from build123d import *

# Parameters (mm, degrees)
SKETCH2_R           = 56.35625
BOSS_EXTRUDE1_DEPTH = 25.4
SKETCH3_R           = 63.5
BOSS_EXTRUDE2_DEPTH = 9.525
SKETCH4_R           = 44.45
CUT_EXTRUDE1_DEPTH  = 97.35484225
SKETCH9_W           = 5.08
SKETCH9_H           = 12.7
FILLET1_R           = 2.54
SKETCH10_R          = 2.54
CUT_EXTRUDE2_DEPTH  = 94.3255592
CIRPATTERN1_COUNT   = 12
HOLE2_START         = 30.099
HOLE2_OUTLINE_R     = 2.413
HOLE2_DEPTH         = 4.826
HOLE2_START_2       = 25.485046345
HOLE2_2_OUTLINE_R   = 1.143
HOLE2_2_DEPTH       = 4.613953655
CIRPATTERN2_COUNT   = 2
HOLE3_D             = 2.286
HOLE3_DEPTH         = 9.438944644
HOLE3_CBORE_D       = 4.826
HOLE3_CBORE_DEPTH   = 4.826
CIRPATTERN3_COUNT   = 2


# Read off the part's stored shape, not the designer's step: Hole2
with BuildPart() as part:
    # Sketch2 → Boss-Extrude1 (new body)
    with BuildSketch(Plane(origin=(0, 0, 0), x_dir=(1, 0, 0), z_dir=(0, 1, 0))):
        with Locations(Location((0, 0, 0), (0, 0, 270))):
            Circle(SKETCH2_R)
    extrude(amount=BOSS_EXTRUDE1_DEPTH)

    # Sketch3 → Boss-Extrude2 (add)
    with BuildSketch(Plane(origin=(0, 25.4, 0), x_dir=(1, 0, 0), z_dir=(0, 1, 0))):
        with Locations(Location((0, 0, 0), (0, 0, 90))):
            Circle(SKETCH3_R)
    extrude(amount=BOSS_EXTRUDE2_DEPTH)

    # Sketch4 → Cut-Extrude1 (cut, through all)
    with BuildSketch(Plane.XZ):
        with Locations(Location((0, 0, 0), (0, 0, 270))):
            Circle(SKETCH4_R)
    extrude(amount=-CUT_EXTRUDE1_DEPTH, mode=Mode.SUBTRACT)

    # Sketch9 → Cut-Revolve1 (revolve, cut)
    with BuildSketch(Plane(origin=(0, 0, 0), x_dir=(0, 0, -1), z_dir=(1, 0, 0))):
        with Locations((53.81625, 19.05)):
            Rectangle(SKETCH9_W, SKETCH9_H)
    revolve(axis=Axis((0, 0, 0), (0, 1, 0)), mode=Mode.SUBTRACT)

    # Fillet1
    fillet1_edges = [part.edges().sort_by_distance(p)[0] for p in [
        (0, 12.7, 51.27625),
        (0, 25.4, 51.27625),
    ]]
    fillet(fillet1_edges, radius=FILLET1_R)

    # Sketch10 → Cut-Extrude2 (cut, through all)
    with BuildSketch(Plane.XZ.offset(-25.4)):
        with Locations(Location((58.42, 0, 0), (0, 0, 270))):
            Circle(SKETCH10_R)
        with Locations(Location((50.593204089, -29.21, 0), (0, 0, 270))):
            Circle(SKETCH10_R)
        with Locations(Location((29.21, -50.593204089, 0), (0, 0, 270))):
            Circle(SKETCH10_R)
        with Locations(Location((0, -58.42, 0), (0, 0, 270))):
            Circle(SKETCH10_R)
        with Locations(Location((-29.21, -50.593204089, 0), (0, 0, 270))):
            Circle(SKETCH10_R)
        with Locations(Location((-50.593204089, -29.21, 0), (0, 0, 270))):
            Circle(SKETCH10_R)
        with Locations(Location((-58.42, 0, 0), (0, 0, 270))):
            Circle(SKETCH10_R)
        with Locations(Location((-50.593204089, 29.21, 0), (0, 0, 270))):
            Circle(SKETCH10_R)
        with Locations(Location((-29.21, 50.593204089, 0), (0, 0, 270))):
            Circle(SKETCH10_R)
        with Locations(Location((0, 58.42, 0), (0, 0, 270))):
            Circle(SKETCH10_R)
        with Locations(Location((29.21, 50.593204089, 0), (0, 0, 270))):
            Circle(SKETCH10_R)
        with Locations(Location((50.593204089, 29.21, 0), (0, 0, 270))):
            Circle(SKETCH10_R)
    extrude(amount=-CUT_EXTRUDE2_DEPTH, mode=Mode.SUBTRACT)

    # Sketch12 → #10-32 Tapped Hole1 (revolve, cut)
    with BuildSketch(Plane(origin=(51.562, 0, 0), x_dir=(0, 0, -1), z_dir=(1, 0, 0))):
        Polygon((0, 0), (0, 10.103317848), (2.0193, 8.89), (2.0193, 1.0287), (3.048, 0), align=None)
    f_10_32_tapped_hole1 = revolve(axis=Axis((51.562, -6.35, 0), (0, 1, 0)), mode=Mode.SUBTRACT)

    # CirPattern1: #10-32 Tapped Hole1 ×12 about axis
    cirpattern1_axis = Axis((0, 0, 0), (0, 1, 0))
    for i in range(1, CIRPATTERN1_COUNT):
        add(f_10_32_tapped_hole1.rotate(cirpattern1_axis, i * 360 / CIRPATTERN1_COUNT), mode=Mode.SUBTRACT)

    # Hole2 outline → Hole2 (cut)
    with BuildSketch(Plane(origin=(0, 0, 0), x_dir=(1, 0, 0), z_dir=(0, 1, 0)).offset(HOLE2_START)):
        with Locations((56.429386772, -15.120208615)):
            Circle(HOLE2_OUTLINE_R)
    hole2 = extrude(amount=HOLE2_DEPTH, mode=Mode.SUBTRACT)

    # Hole2 2 outline → Hole2 2 (cut)
    with BuildSketch(Plane(origin=(0, 0, 0), x_dir=(1, 0, 0), z_dir=(0, 1, 0)).offset(HOLE2_START_2)):
        with Locations((56.429386772, -15.120208615)):
            Circle(HOLE2_2_OUTLINE_R)
    hole2_2 = extrude(amount=HOLE2_2_DEPTH, mode=Mode.SUBTRACT)

    # CirPattern2: Hole2, Hole2 2 ×2 about axis
    cirpattern2_axis = Axis((0, 0, 0), (0, 1, 0))
    add([hole2.rotate(cirpattern2_axis, i * 360 / CIRPATTERN2_COUNT) for i in range(1, CIRPATTERN2_COUNT)], mode=Mode.SUBTRACT)
    add([hole2_2.rotate(cirpattern2_axis, i * 360 / CIRPATTERN2_COUNT) for i in range(1, CIRPATTERN2_COUNT)], mode=Mode.SUBTRACT)

    # Hole3
    with Locations(Plane(origin=(0, 0, 0), x_dir=(-1, 0, 0), z_dir=(0, -1, 0))):
        with Locations((-13.345227604, -49.805067455)):
            hole3 = CounterBoreHole(HOLE3_D / 2, HOLE3_CBORE_D / 2, HOLE3_CBORE_DEPTH, depth=HOLE3_DEPTH)

    # CirPattern3: Hole3 ×2 about axis
    cirpattern3_axis = Axis((0, 0, 0), (0, 1, 0))
    for i in range(1, CIRPATTERN3_COUNT):
        add(hole3.rotate(cirpattern3_axis, i * 360 / CIRPATTERN3_COUNT), mode=Mode.SUBTRACT)


solid = part.part
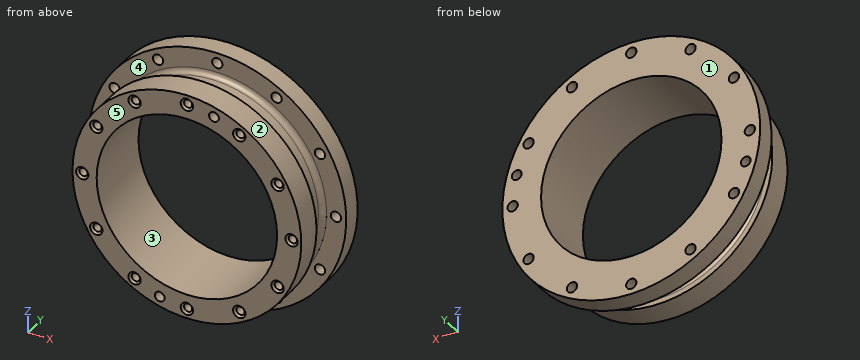
Input: part model. Units: mm. Frame: model coordinates. Face numbers are marked on the shaded views. A direction names the side the tool comes from. Give positions to 0.01 mm unless a question says otherwise; leave off trailing zeros. Write each loop counter-clockwise with the first axis right and the second up, starting at its lowest first coordinate (ties: lowest second). Pieces come first, ordered by that corner, then holes. Notation, with made-up numbers: M 8.5,74.25 L 61.5,74.25 A17 ccw 61.5,85.25 Z; hole C 31.25,55.25 d4. An arc over 180 degrees is marked long. Use one line per item in the form item = value.
1. Ray query, L1, parallel to Z at x = 2, y = 27; L2, parallel to X at y = 29.5, z = -1; L3, parallel to X at y = 7, z = 50.5. Return the intervals inside material, ascending.
Outcome:
L1 = -63.47 to -59.99, -56.85 to -44.4, 44.4 to 56.85, 59.99 to 63.47
L2 = -63.49 to -60.75, -56.09 to -44.44, 44.44 to 56.09, 60.75 to 63.49
L3 = -25.02 to -1.72, 1.72 to 12.44, 14.25 to 25.02
2. Mould query, pull axis X, two halves, no side actions, for the marked faces 1, 2 and 3. Classes: released by +X, released by -X, zero draft, split by the parting line, or undercut.
Outcome:
face_1 = zero draft
face_2 = split by the parting line
face_3 = undercut
3. Cut plane B-B on y = 21. Return loops of the section in (x, z), and give its area (3 significant figures).
Outcome:
outline = C 0,0 d102.55; hole C 0,0 d88.9
area = 2,050 mm²
4. Reachability of the marked faces 4 and 5 from +Z, -Z, +X, -X, +Y, -Y: full face, straight path, thin tool, end or side. Return the list, or none.
Outcome:
face_4 = none
face_5 = +Z, -Z, +X, -X, -Y
5. Cut plane A-A on z = 58.42. Return loops of the section in (x, y) (3 decimals).
Outcome:
outline = M -24.887,25.4 L -2.54,25.4 L -2.54,34.925 L -24.887,34.925 Z; M 2.54,25.4 L 24.887,25.4 L 24.887,34.925 L 2.54,34.925 Z
6. First-contact query: P1, Ø2, axis at x = -50.5, y = 6.5, coming from the -Z side; P2, Ø8, axis at y = 27, z = -40, coming from the -X side; P3, Ø3, axis at y = 3.5, z = -39, coming from the +X side. Flat tips, straight axial feed; report the tip coordinate or a pass-through.
Outcome:
P1 = -26.94
P2 = -52.31
P3 = 42.07
